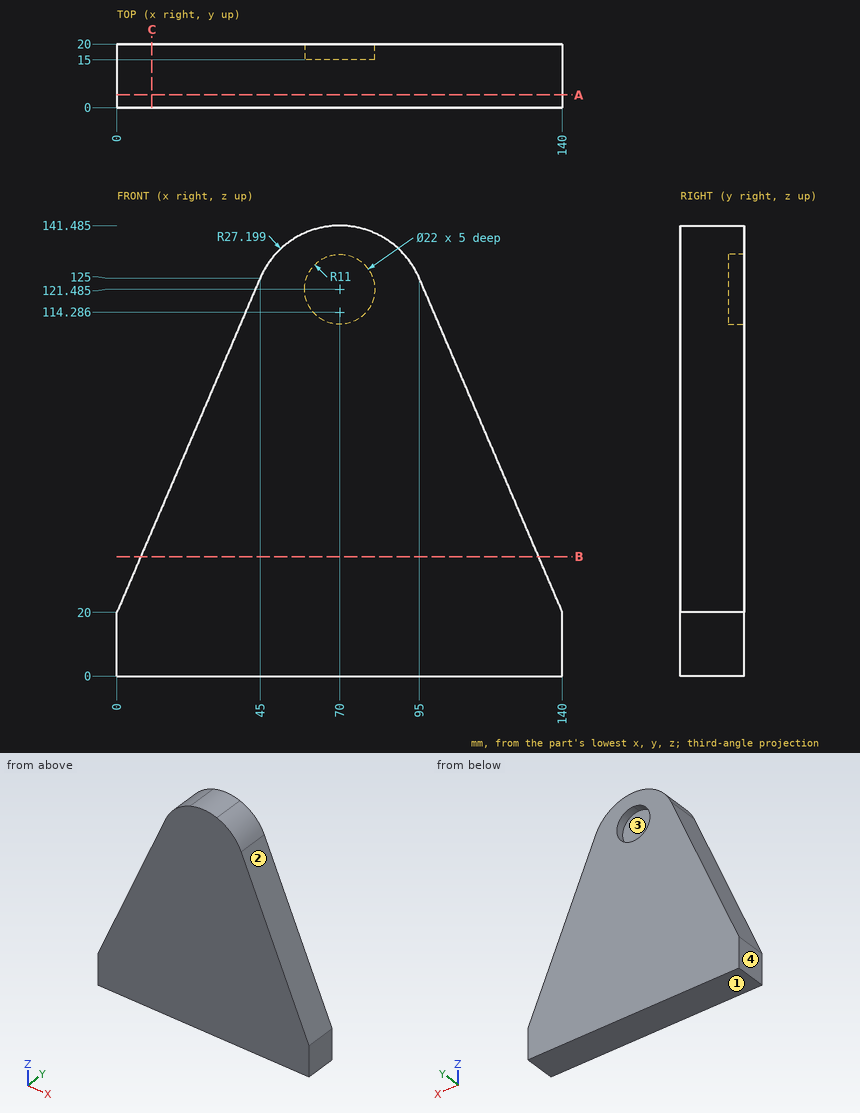
The drawing under review shows one solid part. Ordinate dimensions are in mm from its lowest x, y, z. Coordinates: 2 decimals unless noted, no trailing zeros. Write each loop counter-clockwise with the first axis right and the second up, starting at its lowest first coordinate (ties: lowest second). Pieces come first, ordered by that corner, then holes.
1) Mouldability with a two-part tool opening along X and no side actions: class the marked faces 1, 2, 3 and 4 as +X half, -X half, draft (parallel to the pull), parting line (faces both ways), or undercut.
2) Add section C-C (x = 11). Write out the cut boundary in (y, z).
3) Add section A-A (y = 4). Write out the cut boundary in (x, z), plus the area to 3 significant figures.
4) Add section B-B (z = 37.5). Write out the cut boundary in (x, y).
5) To check wall thickness, follow L1, parallel to Z at x = 70, y = 16.6 (1 decimal); L2, parallel to X at y = 10.5, z = 67; L3, parallel to Z at x = 28, y = 5 (1 decimal). State the ranges of each line that lie inside material, in increasing order.
6) Insertion check: pin 1 (4 mm diameter, centred on x = 102, y = 9, fed in from -Z); pin 2 (17.5 mm diameter, centred on x = 69, z = 121.5, fed in from +Y); pin 3 (5 mm diameter, centred on y = 17, z = 54, fed in from +X); pin 4 (6 mm diameter, centred on y = 16.5, z = 59.5, fed in from +X). Each pin has a flat end and moves straight along its axis. Give the tip position at first contact, or say it passes through.
Check result:
1. face 1: draft
1. face 2: +X half
1. face 3: undercut
1. face 4: -X half
2. outline: (0, 0) - (20, 0) - (20, 45.67) - (0, 45.67) - close
3. outline: (0, 0) - (140, 0) - (140, 20) - (95, 125) arc R27.2 ccw to (45, 125) - (0, 20) - close
3. area: 13,400 mm2
4. outline: (7.5, 0) - (132.5, 0) - (132.5, 20) - (7.5, 20) - close
5. L1: z = 0 to 110.5, 132.5 to 141.5
5. L2: x = 20.14 to 119.86
5. L3: z = 0 to 85.3
6. pin 1: stops at z = 0
6. pin 2: stops at y = 15
6. pin 3: stops at x = 126.5
6. pin 4: stops at x = 124.36
